Geometry: final body of the model. Coordinates: model frame, mm. A direction names the side the tool comes from. Round coordinates to 2 decimals unless told otherwise and drop trailing zeros. Loops run counter-clockwise (first coordinate to the right, second up) from the corner with the lowest first, then second, coordinate; pieces in that order, holes last. Notation, with made-up numbers: (85.25, 28.5) - (102.25, 28.5) arc R17 ccw to (102.25, 61.5) - close; hole circle Ø10 at (59, 89.5). An arc over 180 degrees is marked (long way). Use CSV: the item, a comma, the result in double quotes.
from build123d import *

# Parameters (mm, degrees)
F0_W     = 12.1704526246
F0_H     = 13.7812504545
F0_W_2   = 12.8863714635
F1_DEPTH = 25
F2_W     = 47.6974435151
F2_H     = 21.1193179712
F3_DEPTH = 20
F4_R     = 7.5
F5_DEPTH = 25


with BuildPart() as f1:
    # F0 (on Front) → F1 (new body)
    with BuildSketch(Plane.XZ):
        Polygon((0, 35.3480130434), (0, 0), (55.0355128944, 0), (55.0355128944, 8.5014207289), (42.8650602698, 8.5014207289), (42.8650602698, 22.2826711833), (55.0355128944, 22.2826711833), (55.0355128944, 35.3480130434), align=None)
        with Locations((48.9502865821, 15.3920459561)):
            Rectangle(F0_W, F0_H)
        with Locations((61.4786986262, 15.3920459561)):
            Rectangle(F0_W_2, F0_H)
    extrude(amount=F1_DEPTH)

    # F2 (on face) → F3 (cut)
    with BuildSketch(Plane.XZ.offset(25)):
        with Locations((23.8487217575, 17.2713068314)):
            Rectangle(F2_W, F2_H)
    extrude(amount=-F3_DEPTH, mode=Mode.SUBTRACT)

    # F4 (on face) → F5 (cut)
    with BuildSketch(Plane(origin=(0, 0, 0), x_dir=(-1, 0, 0), z_dir=(0, 1, 0))):
        with Locations((-30, 17.5)):
            Circle(F4_R)
    extrude(amount=-F5_DEPTH, mode=Mode.SUBTRACT)


solid = f1.part
Item 1: Pin query (flat end, axial travel): P1, Ø2, axis at x = 60, y = -10, coming from the +Z side; P2, Ø2, axis at y = -7.5, z = 18.5, coming from the -X side; P3, Ø4.5, axis at y = -16, z = 4.5, coming from the +X side; P4, Ø13.5, axis at x = 30, z = 17.5, coming from the +Y side. Return the tip coordinate at first contact, or that it passes through.
Final values:
P1,"stops at z = 22.28"
P2,"stops at x = 47.7"
P3,"stops at x = 55.04"
P4,"passes through"
Item 2: Section C-C on z = 17.5. Return the cut outline in (x, y), plus the area to 3 significant figures.
Final values:
outline,"(0, -5) - (22.5, -5) - (22.5, 0) - (0, 0) - close; (37.5, -5) - (47.7, -5) - (47.7, -25) - (67.92, -25) - (67.92, 0) - (37.5, 0) - close"
area,"669 mm²"
Item 3: Mould query, pull axis Z, two halves, no side actions, for faces 1 (the flat face through (18, -5, 17)), 2 (the flat face through (61, -12, 8.501)), 3 (the flat face through (67.922, -12, 15)). Classes: released by +Z, released by -Z, zero draft, split by the parting line, or undercut.
Final values:
face 1,"undercut"
face 2,"released by -Z"
face 3,"zero draft"
Item 4: Material intervals for line 1 (Z direction, x = 26.5, y = -20.5); line 2 (Z direction, x = 30, y = -3.35); line 3 (X direction, y = -3.5, z = 34.5), sorted ascending.
Final values:
line 1,"z = 0 to 6.71, 27.83 to 35.35"
line 2,"z = 0 to 10, 25 to 35.35"
line 3,"x = 0 to 55.04"
Item 5: Section A-A on x = 24. Return the cut outline in (y, z), plus the area to 3 significant figures.
Final values:
outline,"(-25, 0) - (0, 0) - (0, 13) - (-5, 13) - (-5, 6.71) - (-25, 6.71) - close; (-25, 27.83) - (-5, 27.83) - (-5, 22) - (0, 22) - (0, 35.35) - (-25, 35.35) - close"
area,"416 mm²"
Item 6: Section B-B on y = -1.75. Return the cut outline in (x, z), plus the area to 3 significant figures.
Final values:
outline,"(0, 0) - (55.04, 0) - (55.04, 8.5) - (67.92, 8.5) - (67.92, 22.28) - (55.04, 22.28) - (55.04, 35.35) - (0, 35.35) - close; hole circle Ø15 at (30, 17.5)"
area,"1,950 mm²"
Item 7: Section D-D on x = 10. Return the cut outline in (y, z).
Final values:
outline,"(-25, 0) - (0, 0) - (0, 35.35) - (-25, 35.35) - (-25, 27.83) - (-5, 27.83) - (-5, 6.71) - (-25, 6.71) - close"
Item 8: Reachability of faces 4 (the flat face through (47.697, -15, 17)), 5 (the flat face through (33, -25, 6)), 6 (the flat face through (55.036, -12, 4)), 7 (the flat face through (55.036, -12, 29)), 8 (the flat face through (28, -12, 35.348)) from +Z, -Z, +X, -X, +Y, -Y: full face, straight path, thin tool, end or side. Return the list, or none.
Final values:
face 4,"-X, -Y"
face 5,"+Z, -Z, +X, -X, -Y"
face 6,"-Z, +X, +Y, -Y"
face 7,"+Z, +X, +Y, -Y"
face 8,"+Z, +X, -X, +Y, -Y"
